```python
from build123d import *

# Parameters (mm, degrees)
SKETCH2_R           = 0.508
BOSS_EXTRUDE1_DEPTH = 0.3175
FILLET1_R           = 0.254
SKETCH3_W           = 1.016
SKETCH3_H           = 1.524
SKETCH3_W_2         = 0.6096
SKETCH3_H_2         = 1.15018662
CUT_EXTRUDE1_DEPTH  = 0.127


with BuildPart() as part:
    # Sketch2 → Boss-Extrude1 (new body, symmetric)
    with BuildSketch(Plane(origin=(0, 0, 0), x_dir=(0, 0, -1), z_dir=(1, 0, 0))):
        with BuildLine():
            Line((0, -0.635), (-116.84, -0.635))
            Line((-116.84, -0.635), (-116.84, 0))
            Line((-116.84, 0), (-0.003451087, 0.634990622))
            ThreePointArc((-0.003451087, 0.634990622), (0.634997655, 0.00172555), (0, -0.635))
        make_face()
        Circle(SKETCH2_R, mode=Mode.SUBTRACT)
    extrude(amount=BOSS_EXTRUDE1_DEPTH, both=True)

    # Fillet1
    fillet1_edges = [part.edges().sort_by_distance(p)[0] for p in [
        (0.3175, -0.3175, 116.84),
        (-0.3175, -0.3175, 116.84),
        (0, -0.635, 116.84),
        (0, 0, 116.84),
    ]]
    fillet(fillet1_edges, radius=FILLET1_R)

    # Sketch3 → Cut-Extrude1 (cut, symmetric)
    with BuildSketch(Plane.XY.offset(12.7)):
        with Locations((0, -0.03450669)):
            Rectangle(SKETCH3_W, SKETCH3_H)
        with Locations((0, -0.03450669)):
            Rectangle(SKETCH3_W_2, SKETCH3_H_2, mode=Mode.SUBTRACT)
    extrude(amount=CUT_EXTRUDE1_DEPTH, both=True, mode=Mode.SUBTRACT)


solid = part.part
```
Here's how the part is built. I have some questions about the finished solid (model axes, mm). Round coordinates to 2 decimals unless told otherwise and drop trailing zeros. Loops run counter-clockwise (first coordinate to the right, second up) from the corner with the lowest first, then second, coordinate; pieces in that order, holes last. Notation, with made-up numbers: (-20, 68.5) -> (-12, 68.5) arc R20 cw to (-12, 81.5) -> close; hole circle Ø3 at (53, 57). An arc over 180 degrees is marked (long way). Answer as CSV lines item,"result".
1. If we section it at C-C on z = 103: Please give me the cut outline in (x, y) (1 decimal), plus the area to 3 significant figures.
Final values:
outline,"(-0.3, -0.6) -> (0.3, -0.6) -> (0.3, 0.1) -> (-0.3, 0.1) -> close"
area,"0.451 mm^2"
2. If we section it at D-D on z = 80: Please give me the cut outline in (x, y) (1 decimal).
Final values:
outline,"(-0.3, -0.6) -> (0.3, -0.6) -> (0.3, 0.2) -> (-0.3, 0.2) -> close"
3. If I drill on L1, parallel to Z at x = 0.1, y = -0.4; L2, parallel to Y at x = 0.2, z = 65 (3 decimals); L3, parallel to Y at x = 0.25, z = 103.5 (1 decimal), over which ranges is the centre line in solid material (lowest first)?
Final values:
L1,"z = -0.49 to -0.31, 0.31 to 116.84"
L2,"y = -0.635 to 0.282"
L3,"y = -0.6 to 0.1"
